```python
from build123d import *

# Parameters (mm, degrees)
SKETCH_1_W          = 41
SKETCH_1_H          = 21
EXTRUDE_1_DEPTH     = 34.9
SKETCH_2_R          = 5.9
SKETCH_2_R_2        = 10.4
EXTRUDE_2_DEPTH     = 4.3
SKETCH_3_R          = 5.75
EXTRUDE_3_DEPTH     = 1.2
SKETCH_4_R          = 3
EXTRUDE_4_DEPTH     = 3.4
SKETCH_5_W          = 2
SKETCH_5_H          = 19
EXTRUDE_5_DEPTH     = 1.5
SKETCH_6_R          = 6.2
EXTRUDE_6_DEPTH     = 2
SKETCH_7_R          = 3
EXTRUDE_7_DEPTH     = 3.5
SKETCH_8_R          = 1
CUT_EXTRUDE_1_DEPTH = 10
SKETCH_9_R          = 5
EXTRUDE_8_DEPTH     = 1
SKETCH_10_R         = 10
EXTRUDE_9_DEPTH     = 2
SKETCH_11_R         = 5
EXTRUDE_10_DEPTH    = 1.6
SKETCH_12_R         = 10
EXTRUDE_11_DEPTH    = 2


with BuildPart() as part:
    # 草圖1 → 填料-伸長1 (new body)
    with BuildSketch(Plane.XY):
        Rectangle(SKETCH_1_W, SKETCH_1_H)
    extrude(amount=EXTRUDE_1_DEPTH)

    # 草圖2 → 填料-伸長2 (add)
    with BuildSketch(Plane(origin=(0, 0, 0), x_dir=(-1, 0, 0), z_dir=(0, 0, -1))):
        with Locations((-1.2, 0)):
            Circle(SKETCH_2_R)
        with Locations((10, 0)):
            Circle(SKETCH_2_R_2)
    extrude(amount=EXTRUDE_2_DEPTH)

    # 草圖3 → 填料-伸長3 (add)
    with BuildSketch(Plane(origin=(0, 0, -4.3), x_dir=(-1, 0, 0), z_dir=(0, 0, -1))):
        with Locations((10, 0)):
            Circle(SKETCH_3_R)
    extrude(amount=EXTRUDE_3_DEPTH)

    # 草圖4 → 填料-伸長4 (add)
    with BuildSketch(Plane(origin=(0, 0, -5.5), x_dir=(-1, 0, 0), z_dir=(0, 0, -1))):
        with Locations((10, 0)):
            Circle(SKETCH_4_R)
    extrude(amount=EXTRUDE_4_DEPTH)

    # 草圖5 → 填料-伸長5 (add)
    with BuildSketch(Plane.ZY.offset(20.5)):
        with Locations((5.7, 0)):
            Rectangle(SKETCH_5_W, SKETCH_5_H)
    extrude_5 = extrude(amount=EXTRUDE_5_DEPTH)

    # 鏡射1: 填料-伸長5 across plane
    add(extrude_5.mirror(Plane(origin=(0, 0, 0), x_dir=(0, 0, 1), z_dir=(1, 0, 0))))

    # 草圖6 → 填料-伸長6 (add)
    with BuildSketch(Plane.XY.offset(34.9)):
        with Locations((-10, 0)):
            Circle(SKETCH_6_R)
    extrude(amount=EXTRUDE_6_DEPTH)

    # 草圖7 → 填料-伸長7 (add)
    with BuildSketch(Plane.XY.offset(36.9)):
        with Locations((-10, 0)):
            Circle(SKETCH_7_R)
    extrude(amount=EXTRUDE_7_DEPTH)

    # 草圖8 → 除料-伸長1 (cut)
    with BuildSketch(Plane.XY.offset(34.9)):
        with Locations((-18, 8)):
            Circle(SKETCH_8_R)
        with Locations((18, 8)):
            Circle(SKETCH_8_R)
        with Locations((18, -8)):
            Circle(SKETCH_8_R)
        with Locations((-18, -8)):
            Circle(SKETCH_8_R)
    extrude(amount=-CUT_EXTRUDE_1_DEPTH, mode=Mode.SUBTRACT)

    # 草圖9 → 填料-伸長8 (add)
    with BuildSketch(Plane.XY.offset(36.9)):
        with Locations((-10, 0)):
            Circle(SKETCH_9_R)
    extrude(amount=EXTRUDE_8_DEPTH)

    # 草圖10 → 填料-伸長9 (add)
    with BuildSketch(Plane.XY.offset(37.9)):
        with Locations((-10, 0)):
            Circle(SKETCH_10_R)
    extrude(amount=EXTRUDE_9_DEPTH)

    # 草圖11 → 填料-伸長10 (add)
    with BuildSketch(Plane(origin=(0, 0, -5.5), x_dir=(-1, 0, 0), z_dir=(0, 0, -1))):
        with Locations((10, 0)):
            Circle(SKETCH_11_R)
    extrude(amount=EXTRUDE_10_DEPTH)

    # 草圖12 → 填料-伸長11 (add)
    with BuildSketch(Plane(origin=(0, 0, -7.1), x_dir=(-1, 0, 0), z_dir=(0, 0, -1))):
        with Locations((10, 0)):
            Circle(SKETCH_12_R)
    extrude(amount=EXTRUDE_11_DEPTH)


solid = part.part
```
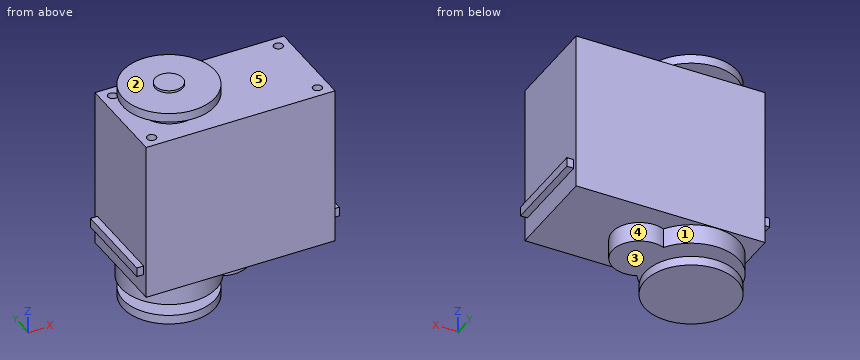
Work out the finished part from the listing and answer in its coordinate system (mm). Face numbers are marked on the shaded views. A direction names the side the tool comes from. Give positions to 0.01 mm unless a question says otherwise; leave off trailing zeros. Loops run counter-clockwise (first coordinate to the right, second up) from the corner with the lowest first, then second, coordinate; pieces in that order, holes last. Notation, with made-up numbers: (26.25, 80) -> (71.25, 80) arc R31 ccw to (71.25, 109) -> close; hole circle Ø5 at (-3, 62.5). An arc over 180 degrees is marked (long way). Put each result on its own line as item: value. Start each with the question number.
Item 1: The part is cut by section C-C (x = 1.2). Give the vertices of the cut face in (y, z).
Item 2: The part is cut by section B-B (x = -18). Give the vertices of the cut face in (y, z), then the cut area to 3 significant figures.
Item 3: Which of the six approach directions +Z, -Z, +X, -X, +Y, -Y give full straight-line access (tool end or side, diameter ignored) to the marked faces 1, 2 and 3?
Item 4: The part is cut by section D-D (z = 17.5). Give the vertices of the cut face in (x, y), then the cut area to 3 significant figures.
Item 5: The part is cut by section A-A (y = 8). State how many separate pieces and enclosed holes the cut face has, then the cut area to 3 significant figures.
Item 6: Each of these flat-tipped pins is pushed along its axis until it touches: P1, Ø1.6, axis at x = -21.5, y = -3, coming from the -Z side; P2, Ø2.5, axis at x = -18, y = -8, coming from the -Z side; P3, Ø1.6, axis at x = -21.5, z = 5, coming from the -Y side. Where does it stop, or does it pass through?
Item 7: Find the intervals of material crossed by L1, parallel to Z at x = -11, y = 7.5; L2, parallel to Y at x = -18, z = 27.75; L3, parallel to Z at x = -7, y = -4.25, in increasing order. Write a range as [from, to].
Item 8: The mould has two halves that part along X. Classify the marked faces 4 and 5: released by +X, released by -X, zero draft, split by the parting line, or undercut.
Answers below:
1. outline: (-10.5, 0) -> (-5.9, 0) -> (-5.9, -4.3) -> (5.9, -4.3) -> (5.9, 0) -> (10.5, 0) -> (10.5, 34.9) -> (-10.5, 34.9) -> close
2. outline: (-10.5, 0) -> (-6.65, 0) -> (-6.65, -4.3) -> (6.65, -4.3) -> (6.65, 0) -> (10.5, 0) -> (10.5, 34.9) -> (9, 34.9) -> (9, 24.9) -> (7, 24.9) -> (7, 34.9) -> (-7, 34.9) -> (-7, 24.9) -> (-9, 24.9) -> (-9, 34.9) -> (-10.5, 34.9) -> close; (-6, -9.1) -> (6, -9.1) -> (6, -7.1) -> (-6, -7.1) -> close; (-6, 37.9) -> (6, 37.9) -> (6, 39.9) -> (-6, 39.9) -> close
2. area: 798 mm2
3. face 1: -Z
3. face 2: +Z
3. face 3: none
4. outline: (-20.5, -10.5) -> (20.5, -10.5) -> (20.5, 10.5) -> (-20.5, 10.5) -> close
4. area: 861 mm2
5. separate pieces: 3
5. enclosed holes: 0
5. area: 1,500 mm2
6. P1: z = 4.7
6. P2: z = -4.3
6. P3: y = -9.5
7. L1: [-9.1, -7.1], [-4.3, 34.9], [37.9, 39.9]
7. L2: [-10.5, -9], [-7, 7], [9, 10.5]
7. L3: [-9.1, -7.1], [-5.5, 36.9], [37.9, 39.9]
8. face 4: undercut
8. face 5: zero draft
